Answer from the drawing. Dimensions are ordinates in mm from the lowest x, y and z of the part. A direction names the side the tool comes from. Coordinates: 2 decimals unless noted, no trailing zeros. Write each loop counter-clockwise with the first axis right and the second up, starting at its lowest first coordinate (ties: lowest second). Pieces come first, ordered by that corner, then holes. Notation, with made-up numbers: (81, 11.5) -> (85, 11.5) arc R16 ccw to (85, 25.5) -> close; hole circle Ø2 at (9, 67). An arc over 180 degrees is marked (long way). Return JSON: item names as keys, results as strings.
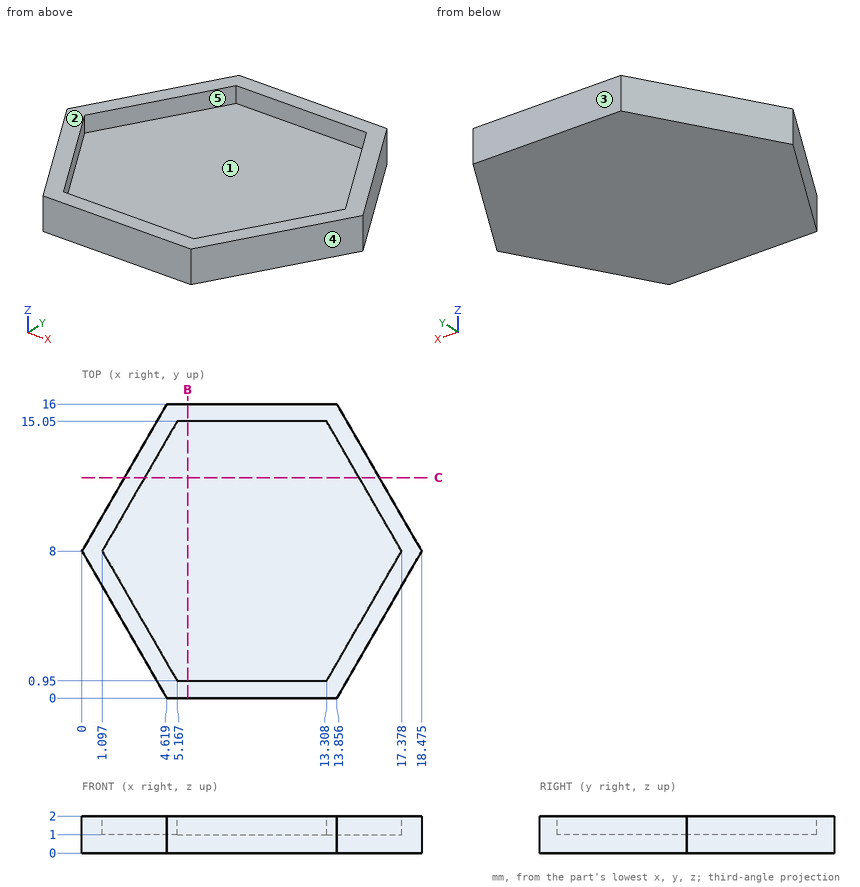
1. Consider L1, parallel to Y at x = 6.5, z = 1.6; L2, parallel to Z at x = 10, y = 14; L3, parallel to X at y = 6.25, z = 1.45 (1 decimal). Determine where each line is inside the solid, lowest interval first.
Taken from the geometry:
{"L1": "y = 0 to 0.95, 15.05 to 16", "L2": "z = 0 to 1", "L3": "x = 1 to 2.1, 16.4 to 17.5"}
2. A flat-ended cylindrical pin translates along its axis: pin 1 Ø1 at (x, y) = (6.5, 10.5) entering from +Z. Find the tip coordinate at first contact, or state that the pin passes through.
Taken from the geometry:
{"pin 1": "stops at z = 1"}
3. A tool of negligible diameter and unlimited length cuts with its end or side. For the marked faces 4 and 5, from which of +Z, -Z, +X, -X, +Y, -Y can it reach the whole face along a straight path? Write none if from no direction.
Taken from the geometry:
{"face 4": "+Z, -Z, +X, -Y", "face 5": "+Z"}
4. For a pull along Y with two mould halves and no side action, classify the marked faces 1, 2 and 3 as +Y half, -Y half, draft (parallel to the pull), parting line (faces both ways), or undercut.
Taken from the geometry:
{"face 1": "undercut", "face 2": "draft", "face 3": "+Y half"}
5. The part is cut by section C-C (y = 12). Determine the outline of the cut face in (x, z) (1 decimal).
Taken from the geometry:
{"outline": "(2.3, 0) -> (16.2, 0) -> (16.2, 2) -> (15.1, 2) -> (15.1, 1) -> (3.4, 1) -> (3.4, 2) -> (2.3, 2) -> close"}
6. The part is cut by section B-B (x = 5.75). Determine the outline of the cut face in (y, z).
Taken from the geometry:
{"outline": "(0, 0) -> (16, 0) -> (16, 2) -> (15.05, 2) -> (15.05, 1) -> (0.95, 1) -> (0.95, 2) -> (0, 2) -> close"}
